Geometry: final body of the model. Coordinates: model frame, mm. Face numbers are marked on the shaded views. Give positions to 0.01 mm unless a question says otherwise; leave off trailing zeros. Order: outer loops, then holes, each group sorted by start corner. A loop starts at its lowest first (then second) coordinate and runs counter-clockwise, first axis right, second up. Notation, with made-up numbers: (19, 46.25) - (32, 46.25) arc R22 cw to (32, 54.25) - close; hole circle Ø5 at (58.5, -16.5). An arc over 180 degrees is marked (long way). Put each result on its own line as item: value. Start each with the question number.
1. Section C-C on z = 196.5. Return the cut outline in (x, y).
2. Ray query, line 1 along X through (y, z) = (-344.5, 0) (3 decimals); line 2 along X through (y, z) = (-262, -4.5). Return the intervals inside material, ascending. Write a range as from..to.
3. First-contact query: P1, Ø1, axis at y = -343, z = 91, coming from the +X side; P2, Ø15, axis at x = 316.5, z = -40, coming from the +Y side; P3, Ø19.5, axis at x = 293.5, y = -157, coming from the -Z side. Flat tips, straight axial feed; report the tip coordinate or a pass-through.
4. Section A-A on z = 0. Return the cut outline in (x, y) (3 decimals).
5. Mould query, pull axis X, two halves, no side actions, for the marked faces 1, 2 and 3. Classes: pulls with the +X half, pulls with the -X half, needs draft (parallel to the pull), parting line crosses it, or undercut.
from build123d import *

# Parameters (mm, degrees)
F0_R        = 323.85
F0_R_2      = 320.675
F1_DEPTH    = 469.9
F2_W        = 298.45
F2_H        = 298.45
F3_DEPTH    = 595.884
F5_DEPTH    = 612.14
F6_T4_ANGLE = 57.0256517653
F7_R        = 669.2625565618
F7_R_2      = 339.725
F7_R_3      = 320.675
F8_DEPTH    = 561.34
F10_DEPTH   = 323.85
F11_R       = 104.775
F12_DEPTH   = 947.42
F13_DEPTH   = 20.32


# Not quite as in the source:
# - a fillet or chamfer that OpenCascade refuses, or shapes differently, is made with other operations: its cross-section is extruded or revolved along the edge and cut away or added


with BuildPart() as f1:
    # F0 (on Front) → F1 (new body)
    with BuildSketch(Plane.XZ):
        Circle(F0_R)
        Circle(F0_R_2, mode=Mode.SUBTRACT)
    extrude(amount=F1_DEPTH)

    # F2 (on Right) → F3 (cut)
    with BuildSketch(Plane.YZ):
        with Locations((-149.225, 0)):
            Rectangle(F2_W, F2_H)
    extrude(amount=F3_DEPTH, mode=Mode.SUBTRACT)

    # F4 (on Right) → F5 (join)
    with BuildSketch(Plane.YZ):
        Polygon((20.32, 149.225), (0, 149.225), (-323.85, 149.225), (-323.85, -149.225), (0, -149.225), (20.32, -149.225), (20.32, -144.145), (0, -144.145), (-17.1384390951, -144.145), (-306.7115609049, -144.145), (-306.7115609049, 144.145), (-17.1384390951, 144.145), (0, 144.145), (20.32, 144.145), align=None)
    extrude(amount=F5_DEPTH)

    # F6: fillet of radius 5.08 on 1 edges, made by hand


with BuildPart() as f6_tool2:
    # F6_s3 → F6_t4 (revolve)
    with BuildSketch(Plane(origin=(0, 0, 0), x_dir=(0, 1, 0), z_dir=(-0.4773554749, 0, 0.8787102768))):
        with BuildLine():
            ThreePointArc((-303.1592860393, -323.85), (-300.3194797079, -322.9821134838), (-298.45, -320.675))
            Line((-298.45, -320.675), (-298.45, -323.85))
            Line((-298.45, -323.85), (-303.1592860393, -323.85))
        make_face()
    revolve(axis=Axis((0, -298.45, 0), (0, 1, 0)), revolution_arc=F6_T4_ANGLE)

    split(bisect_by=Plane.XY.offset(-144.145), keep=Keep.TOP)

    split(bisect_by=Plane.XY.offset(144.145), keep=Keep.BOTTOM)


with BuildPart() as f1_1:
    add(f1.part)

    # F6_t1: cut F6_tool2
    add(f6_tool2.part, mode=Mode.SUBTRACT)

    # F7 (on Front) → F8 (cut, symmetric)
    with BuildSketch(Plane.XZ):
        Circle(F7_R)
        Circle(F7_R_2, mode=Mode.SUBTRACT)
        Circle(F7_R_3)
    extrude(amount=F8_DEPTH, both=True, mode=Mode.SUBTRACT)

    # F9 (on Front) → F10 (join, through all)
    with BuildSketch(Plane.XZ):
        with BuildLine():
            ThreePointArc((305.1966169537, 149.225), (339.725, 0), (305.1966169537, -149.225))
            Line((305.1966169537, -149.225), (308.0214758747, -149.225))
            ThreePointArc((308.0214758747, -149.225), (342.265, 0), (308.0214758747, 149.225))
            Line((308.0214758747, 149.225), (305.1966169537, 149.225))
        make_face()
    extrude(amount=F10_DEPTH)

    # F11 (on Right) → F12 (cut)
    with BuildSketch(Plane.YZ):
        with Locations((-136.525, 0)):
            Circle(F11_R)
    extrude(amount=F12_DEPTH, mode=Mode.SUBTRACT)

    # F9 (on Front) → F13 (join)
    with BuildSketch(Plane.XZ):
        with BuildLine():
            ThreePointArc((305.1966169537, 149.225), (339.725, 0), (305.1966169537, -149.225))
            Line((305.1966169537, -149.225), (308.0214758747, -149.225))
            ThreePointArc((308.0214758747, -149.225), (342.265, 0), (308.0214758747, 149.225))
            Line((308.0214758747, 149.225), (305.1966169537, 149.225))
        make_face()
    extrude(amount=-F13_DEPTH)


solid = f1_1.part
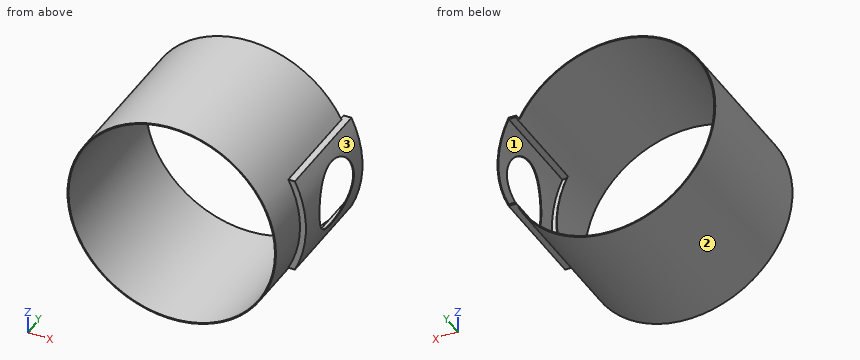
Resolved:
1. outline: (-257.42, -469.9) - (-253.42, -469.9) - (-253.42, 0) - (-257.42, 0) - close; (253.42, -469.9) - (257.42, -469.9) - (257.42, 0) - (253.42, 0) - close
2. line 1: -323.85..-320.675, 320.675..323.85
2. line 2: -323.82..-320.64, 339.7..342.24
3. P1: x = 310.95
3. P2: y = -298.45
3. P3: z = -156.09
4. outline: (-323.85, -469.9) - (-320.675, -469.9) - (-320.675, 0) - (-323.85, 0) - close; (320.675, -469.9) - (323.85, -469.9) - (323.85, -323.85) - (342.265, -323.85) - (342.265, -241.3) - (339.725, -241.3) - (339.725, -306.712) - (323.85, -306.712) - (323.85, -303.159) arc R5.08 ccw to (320.675, -298.45) - close; (339.725, -31.75) - (342.265, -31.75) - (342.265, 20.32) - (339.725, 20.32) - close
5. face 1: undercut
5. face 2: parting line crosses it
5. face 3: pulls with the +X half
